```python
from build123d import *

# Parameters (mm, degrees)
SKETCH1_W              = 26
SKETCH1_H              = 36
BOSS_EXTRUDE1_DEPTH    = 10
BOSS_EXTRUDE2_DEPTH    = 7
FILLET1_R              = 2
SPLIT1_SURFACE_1_BACK  = 48.55
SPLIT1_SURFACE_1_DEPTH = 97.1


with BuildPart() as part:
    # Sketch1 → Boss-Extrude1 (new body)
    with BuildSketch(Plane(origin=(0, 0, 0), x_dir=(1, 0, 0), z_dir=(0, 1, 0))):
        Rectangle(SKETCH1_W, SKETCH1_H)
    extrude(amount=BOSS_EXTRUDE1_DEPTH)

    # Sketch2 → Boss-Extrude2 (add)
    with BuildSketch(Plane(origin=(0, 10, 0), x_dir=(1, 0, 0), z_dir=(0, 1, 0))):
        with BuildLine():
            Line((10, 18), (10, -4.5))
            ThreePointArc((10, -4.5), (0, -14.5), (-10, -4.5))
            Line((-10, -4.5), (-10, 18))
            Line((-10, 18), (10, 18))
        make_face()
    extrude(amount=BOSS_EXTRUDE2_DEPTH)

    # Fillet1
    fillet1_edges = [part.edges().sort_by_distance(p)[0] for p in [
        (-10, 10, -6.75),
        (0, 10, 14.5),
        (10, 10, -6.75),
    ]]
    fillet(fillet1_edges, radius=FILLET1_R)

    # Split1: cut with a surface, the side it looks to stays
    # Split1 surface: a surface, the sketch's curves swept straight by 97.1 mm
    with BuildLine(Plane.XY.offset(18).offset(-SPLIT1_SURFACE_1_BACK), mode=Mode.PRIVATE) as split1_surface_1_path:
        Line((-13, 10), (13, 10))
    split1_surface_1 = Shell.extrude(split1_surface_1_path.wire(), (0 * SPLIT1_SURFACE_1_DEPTH, 0 * SPLIT1_SURFACE_1_DEPTH, 1 * SPLIT1_SURFACE_1_DEPTH))
    split(bisect_by=split1_surface_1, keep=Keep.TOP)

    # Mirror1: part across plane


with BuildPart() as part_1:
    add(part.part)
    add(part.part.mirror(Plane(origin=(13, 10, -18), x_dir=(1, 0, 0), z_dir=(0, 0, 1))))


solid = part_1.part
```
The listing builds one solid part. Answer for the finished solid, in the listing's coordinates (mm). A direction names the side the tool comes from. Give positions to 0.01 mm unless a question says otherwise; leave off trailing zeros. Order: outer loops, then holes, each group sorted by start corner. A loop starts at its lowest first (then second) coordinate and runs counter-clockwise, first axis right, second up.
1) Given P1, Ø4, axis at x = 5, y = 14.5, coming from the -Z side; P2, Ø2.5, axis at y = 14.5, z = -13, coming from the -X side; P3, Ø2.5, axis at y = 14, z = -26, coming from the +X side, each flat-ended and moving along its own axis, determine where each tip first touches the part or whether it passes through.
Reported:
P1: stops at z = -50.04
P2: stops at x = -10
P3: stops at x = 10
2) For faces 1 (the face through (10, 14, -18)), 2 (the face through (-10, 14, -18)), 3 (the face through (0.2, 14.5, -50.5)), determine the directions among +Z, -Z, +X, -X, +Y, -Y from which every point of the face is accessible in a straight line to the end or side of a thin tool.
Reported:
face 1: +Z, -Z, +X, +Y
face 2: +Z, -Z, -X, +Y
face 3: -Z, +Y
3) Consider line 1 along X through (y, z) = (12.75, -31); line 2 along Y through (x, z) = (-10.25, 3); line 3 along Z through (x, y) = (-3.25, 14.25). Determine where each line is inside the solid, lowest interval first.
Reported:
line 1: x = -10 to 10
line 2: y = 10 to 11.03
line 3: z = -49.96 to 13.96
4) Find section C-C on y = 15.25. Write down the section's boundary in (x, z).
Reported:
outline: (-10, -40.5) arc R10 ccw to (10, -40.5) - (10, 4.5) arc R10 ccw to (-10, 4.5) - close
5) Find section B-B on z = -39. Write down the section's boundary in (x, y), then the cut area to 3 significant figures.
Reported:
outline: (-12, 10) - (12, 10) arc R2 cw to (10, 12) - (10, 17) - (-10, 17) - (-10, 12) arc R2 cw to start
area: 142 mm2
6) Find section A-A on x = 0. Write down the section's boundary in (y, z).
Reported:
outline: (10, -52.5) arc R2 cw to (12, -50.5) - (17, -50.5) - (17, 14.5) - (12, 14.5) arc R2 cw to (10, 16.5) - close
